For this review, use the dimensioned drawing (mm, ordinates from the lowest corner) and the shaded views. A direction names the side the tool comes from. Give positions to 0.01 mm unless a question says otherwise; leave off trailing zeros. Loops run counter-clockwise (first coordinate to the right, second up) from the corner with the lowest first, then second, coordinate; pieces in that order, holes last. Notation, with made-up numbers: (-27, -27) -> (25, -27) arc R23 cw to (25, -17) -> close; hole circle Ø7 at (2.25, 13.5). An arc over 180 degrees is marked (long way). Write each question's results on one line, items separated by ' | '. Start each with the question number.
Q1. We need section B-B (x = 19). Write out the cut boundary in (y, z).
Q2. We need section A-A (y = 3.6). Write out the cut boundary in (x, z) (1 decimal), plus the area to 3 significant figures.
Q3. Machinability: for the marked faces 1, 2, 3, 4 and 5, which of the approach directions +Z, -Z, +X, -X, +Y, -Y give a long, thin tool a straight path to every point of the face, cutting with its end or side? Answer none if there is none.
Q4. Insertion check: pin 1 Ø18.5 at (x, z) = (22.22, 22.48) entering from +Y; pin 2 Ø3 at (y, z) = (5, 7.5) entering from +X; pin 3 Ø2.5 at (y, z) = (5, 23) entering from -X; pin 4 Ø3 at (x, z) = (6.5, 16.5) entering from +Y. Each pin has a flat end and moves straight along its axis. Give the tip position at first contact, or say it passes through.
Q5. Wall thickness on L1, parallel to Y at x = 27.5, z = 11.5; L2, parallel to X at y = 1.4, z = 26.5 (1 decimal); L3, parallel to Z at x = 17.5, y = 2.1 (1 decimal): over which ranges is each line inside the solid? List them lowest first. Write a range as [from, to].
Q6. We need section D-D (x = 7). Write out the cut boundary in (y, z) (1 decimal).
Q7. We need section C-C (z = 30). Write out the cut boundary in (x, y), plus the area to 3 significant figures.
Q8. Mouldability with a two-part tool opening along X and no side actions: class the marked faces 6, 7 and 8 as released by +X, released by -X, zero draft, split by the parting line, or undercut.
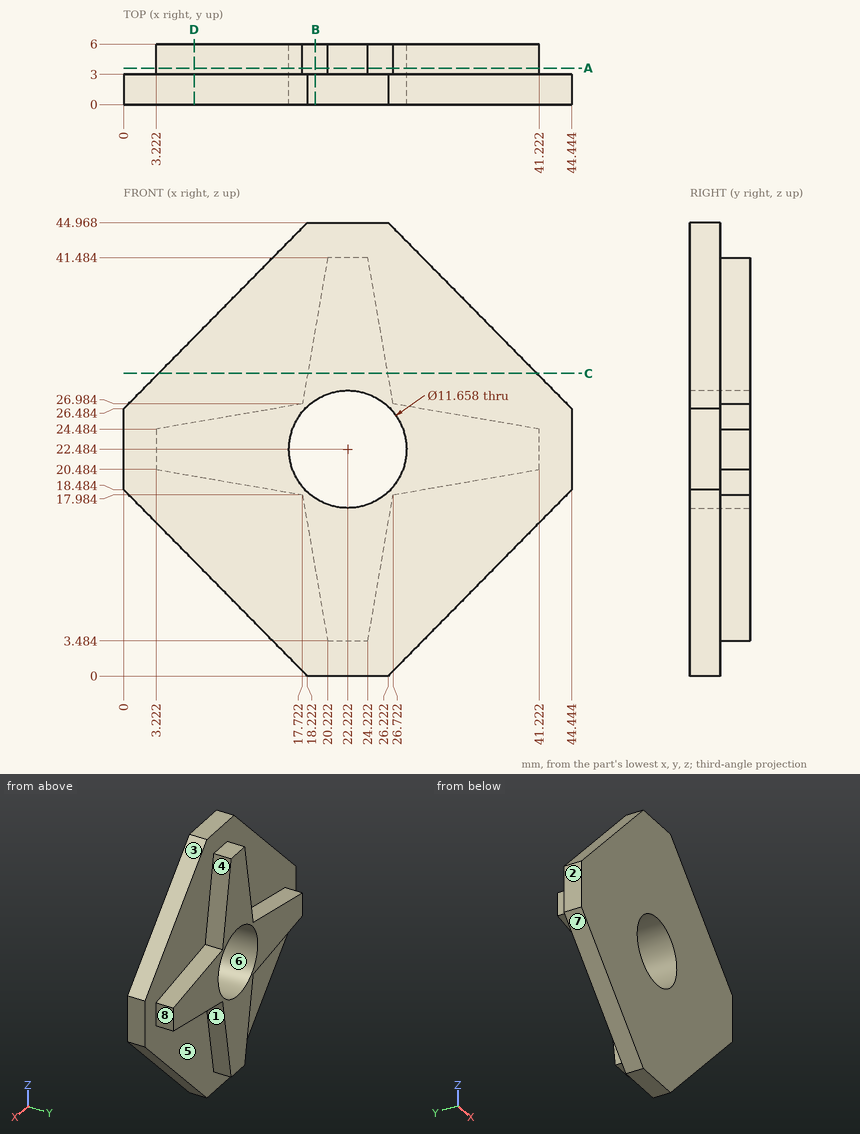
Output:
1) outline: (0, 0) -> (3, 0) -> (3, 10.57) -> (6, 10.57) -> (6, 17.63) -> (0, 17.63) -> close; (0, 27.34) -> (6, 27.34) -> (6, 34.4) -> (3, 34.4) -> (3, 44.97) -> (0, 44.97) -> close
2) outline: (3.2, 20.5) -> (17.7, 18) -> (20.2, 3.5) -> (24.2, 3.5) -> (26.7, 18) -> (41.2, 20.5) -> (41.2, 24.5) -> (26.7, 27) -> (24.2, 41.5) -> (20.2, 41.5) -> (17.7, 27) -> (3.2, 24.5) -> close; hole circle Ø11.7 at (22.2, 22.5) | area: 351 mm2
3) face 1: -Z, +X, +Y | face 2: +Z, -Z, -X, +Y, -Y | face 3: +Z, +X, +Y, -Y | face 4: +Z, +X, +Y | face 5: +Y
4) pin 1: y = 6 | pin 2: x = 25.17 | pin 3: x = 3.22 | pin 4: y = 3
5) L1: [0, 3] | L2: [0, 18], [26.4, 44.4] | L3: [0.7, 19.1], [25.9, 44.2]
6) outline: (0, 11.4) -> (3, 11.4) -> (3, 19.8) -> (6, 19.8) -> (6, 25.1) -> (3, 25.1) -> (3, 33.6) -> (0, 33.6) -> close
7) outline: (3.47, 0) -> (40.98, 0) -> (40.98, 3) -> (26.2, 3) -> (26.2, 6) -> (18.24, 6) -> (18.24, 3) -> (3.47, 3) -> close | area: 136 mm2
8) face 6: undercut | face 7: released by -X | face 8: released by +X
